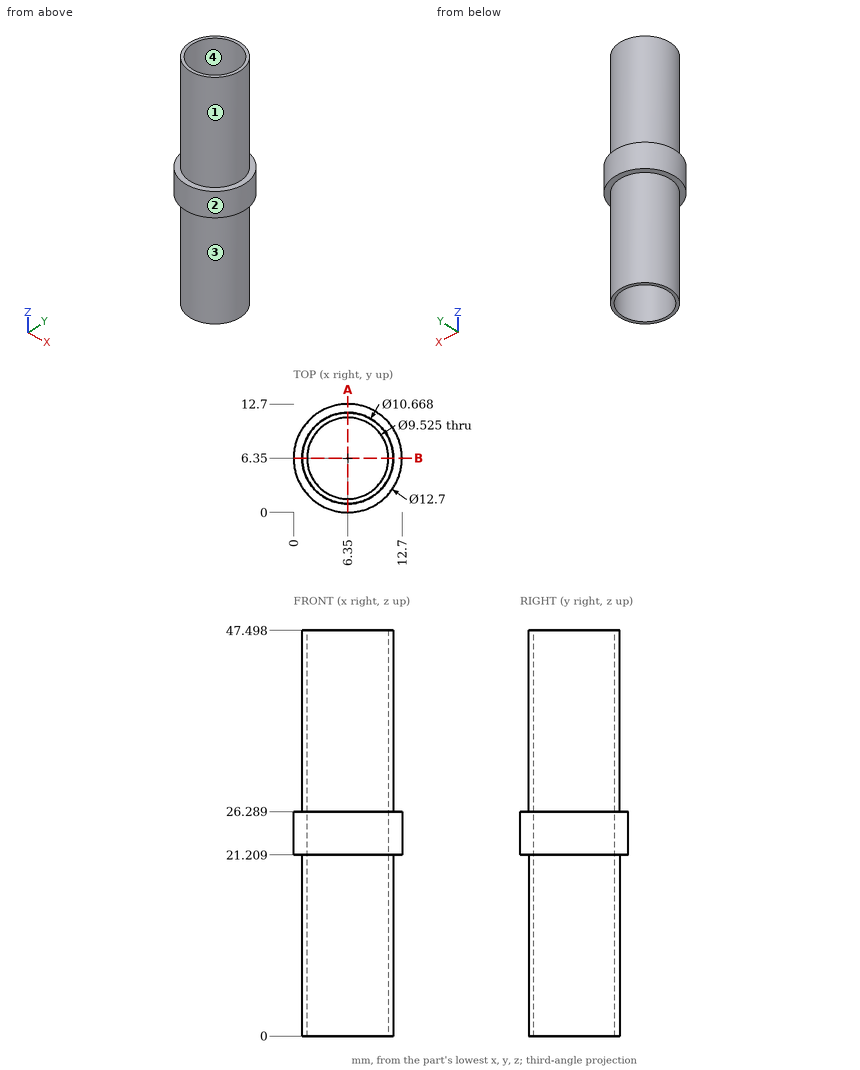
Study the drawing (mm; zero at the part's minimum x, y, z) and answer. A direction names the side the tool comes from. Give positions to 0.01 mm unless a question says otherwise; leave off trailing zeros. Loops run counter-clockwise (first coordinate to the right, second up) from the corner with the lowest first, then second, coordinate; pieces in that order, holes last. Notation, with made-up numbers: M -29.75,89 L -18.75,89 A5 cw -18.75,96 Z; hole C -3,50.5 d7. An arc over 180 degrees is marked long. One line per item, written item: value. Start each with the question number.
1. This flat-tipped pin is pushed along its axis until it touches: P1, Ø1, axis at x = 10, z = 42, coming from the -Y side. Where does it stop, or does it pass through?
2. Find section A-A (x = 6.35). Give the vertices of the cut face in (y, z).
3. Determine the mould class of the marked faces 3 and 4 for opening direction X: released by +X, released by -X, zero draft, split by the parting line, or undercut.
4. Which of the six approach directions +Z, -Z, +X, -X, +Y, -Y give full straight-line access (tool end or side, diameter ignored) to the marked faces 1 and 2?
5. Find the intervals of material crossed by probe 1 along Y at (x, z) = (6.35, 19.5); probe 2 along Z at (x, y) = (1, 7.75); probe 3 along Y at (x, z) = (8.5, 37), in increasing order.
Reported:
1. P1: stops at y = 2.05
2. outline: M 0,21.21 L 1.02,21.21 L 1.02,0 L 1.59,0 L 1.59,47.5 L 1.02,47.5 L 1.02,26.29 L 0,26.29 Z; M 11.11,0 L 11.68,0 L 11.68,21.21 L 12.7,21.21 L 12.7,26.29 L 11.68,26.29 L 11.68,47.5 L 11.11,47.5 Z
3. face 3: split by the parting line
3. face 4: undercut
4. face 1: +Z
4. face 2: +Z, -Z
5. probe 1: y = 1.02 to 1.59, 11.11 to 11.68
5. probe 2: z = 21.21 to 26.29
5. probe 3: y = 1.47 to 2.1, 10.6 to 11.23
